from build123d import *

# Parameters (mm, degrees)
EXTRUDE_1_DEPTH     = 22.7
CUT_EXTRUDE_1_DEPTH = 1.2
SKETCH_3_R          = 1.25
SKETCH_3_W          = 8
SKETCH_3_H          = 6
CUT_EXTRUDE_2_DEPTH = 5
SKETCH_4_R          = 0.75
CUT_EXTRUDE_3_DEPTH = 5


with BuildPart() as part:
    # 草图1 → 凸台-拉伸1 (new body)
    with BuildSketch(Plane.XY):
        with BuildLine():
            Line((1.5, 0), (26.5, 0))
            ThreePointArc((26.5, 0), (27.560660172, 0.439339828), (28, 1.5))
            Line((28, 1.5), (28, 12.1))
            ThreePointArc((28, 12.1), (27.560660172, 13.160660172), (26.5, 13.6))
            Line((26.5, 13.6), (1.5, 13.6))
            ThreePointArc((1.5, 13.6), (0.439339828, 13.160660172), (0, 12.1))
            Line((0, 12.1), (0, 1.5))
            ThreePointArc((0, 1.5), (0.439339828, 0.439339828), (1.5, 0))
        make_face()
    extrude(amount=EXTRUDE_1_DEPTH)

    # 草图2 → 切除-拉伸1 (cut)
    with BuildSketch(Plane.XY.offset(22.7)):
        with BuildLine():
            ThreePointArc((0, 6.800000018), (1.991673894, 11.608326118), (6.8, 13.6))
            Line((6.8, 13.6), (1.5, 13.6))
            ThreePointArc((1.5, 13.6), (0.439339828, 13.160660172), (0, 12.1))
            Line((0, 12.1), (0, 6.800000018))
        make_face()
        with BuildLine():
            ThreePointArc((6.8, 0), (1.991673882, 1.991673894), (0, 6.800000018))
            Line((0, 6.800000018), (0, 1.5))
            ThreePointArc((0, 1.5), (0.439339828, 0.439339828), (1.5, 0))
            Line((1.5, 0), (6.8, 0))
        make_face()
        with BuildLine():
            Line((28, 1.5), (28, 6.8))
            ThreePointArc((28, 6.8), (26.008326112, 1.991673888), (21.2, 0))
            Line((21.2, 0), (26.5, 0))
            ThreePointArc((26.5, 0), (27.560660172, 0.439339828), (28, 1.5))
        make_face()
        with BuildLine():
            Line((26.5, 13.6), (21.2, 13.6))
            ThreePointArc((21.2, 13.6), (26.008326112, 11.608326112), (28, 6.8))
            Line((28, 6.8), (28, 12.1))
            ThreePointArc((28, 12.1), (27.560660172, 13.160660172), (26.5, 13.6))
        make_face()
    extrude(amount=-CUT_EXTRUDE_1_DEPTH, mode=Mode.SUBTRACT)

    # 草图3 → 切除-拉伸2 (cut)
    with BuildSketch(Plane(origin=(0, 0, 0), x_dir=(-1, 0, 0), z_dir=(0, 0, -1))):
        with Locations((-24.8, 6.8)):
            Circle(SKETCH_3_R)
        with Locations((-3.2, 6.8)):
            Circle(SKETCH_3_R)
        with Locations((-14, 6.8)):
            Rectangle(SKETCH_3_W, SKETCH_3_H)
    extrude(amount=-CUT_EXTRUDE_2_DEPTH, mode=Mode.SUBTRACT)

    # 草图4 → 切除-拉伸3 (cut)
    with BuildSketch(Plane.XZ):
        with Locations((24.8, 11.6)):
            Circle(SKETCH_4_R)
        with Locations((3.2, 11.6)):
            Circle(SKETCH_4_R)
    extrude(amount=-CUT_EXTRUDE_3_DEPTH, mode=Mode.SUBTRACT)


solid = part.part
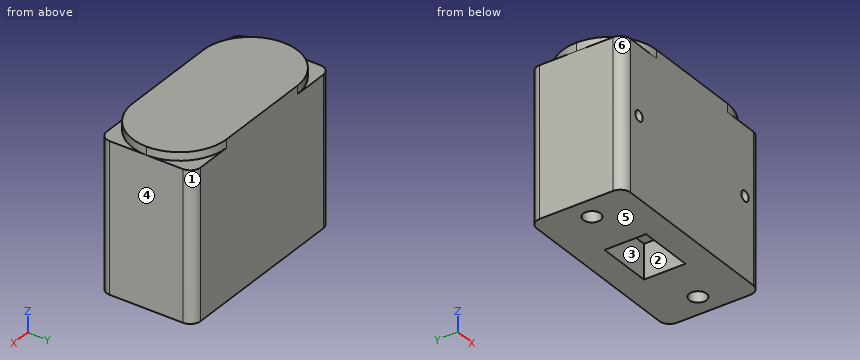
The listing builds one solid part. Answer for the finished solid, in the listing's coordinates (mm). Face numbers are marked on the shaded views. A direction names the side the tool comes from. Coordinates: 2 decimals unless noted, no trailing zeros. Write each loop counter-clockwise with the first axis right and the second up, starting at its lowest first coordinate (ties: lowest second). Pieces come first, ordered by that corner, then holes. Notation, with made-up numbers: (41, 36) - (76, 36) arc R23 cw to (76, 50) - close; hole circle Ø3 at (-6.5, 67.5). An arc over 180 degrees is marked (long way). Put each result on its own line as item: value.
1. The part is cut by section B-B on z = 11.6. Give the vertices of the cut face in (x, y).
Answer sheet:
outline: (0, 1.5) arc R1.5 ccw to (1.5, 0) - (2.45, 0) - (2.45, 5) - (3.95, 5) - (3.95, 0) - (24.05, 0) - (24.05, 5) - (25.55, 5) - (25.55, 0) - (26.5, 0) arc R1.5 ccw to (28, 1.5) - (28, 12.1) arc R1.5 ccw to (26.5, 13.6) - (1.5, 13.6) arc R1.5 ccw to (0, 12.1) - close
2. Determine the mould class of the marked faces 3, 4, 5 and 6 for opening direction X: pulls with the +X half, pulls with the -X half, needs draft (parallel to the pull), parting line crosses it, or undercut.
Answer sheet:
face 3: undercut
face 4: pulls with the +X half
face 5: needs draft
face 6: pulls with the -X half
3. The part is cut by section D-D on x = 3.2. Give the vertices of the cut face in (y, z), plus the area to 3 significant figures.
Answer sheet:
outline: (0, 0) - (5.55, 0) - (5.55, 5) - (8.05, 5) - (8.05, 0) - (13.6, 0) - (13.6, 21.5) - (12.57, 21.5) - (12.57, 22.7) - (1.03, 22.7) - (1.03, 21.5) - (0, 21.5) - (0, 12.35) - (5, 12.35) - (5, 10.85) - (0, 10.85) - close
area: 286 mm^2
4. Find the intervals of material crossed by line 1 along Z through (x, y) = (24.8, 2.25); line 2 along Y through (x, z) = (24.8, 2.45); line 3 along X through (y, z) = (12.25, 16.5), in increasing order. Write a range as from..to.
Answer sheet:
line 1: z = 0..10.85, 12.35..22.7
line 2: y = 0..5.55, 8.05..13.6
line 3: x = 0.01..27.99
5. A tool of negligible diameter and unlimited length cuts with its end or side. For the marked faces 1 and 2, from which of +Z, -Z, +X, -X, +Y, -Y can it reach the whole face along a straight path? Write none if from no direction.
Answer sheet:
face 1: +Z, -Z, +X, +Y
face 2: -Z
6. The part is cut by section A-A on x = 13.25. Give the vertices of the cut face in (y, z).
Answer sheet:
outline: (0, 0) - (3.8, 0) - (3.8, 5) - (9.8, 5) - (9.8, 0) - (13.6, 0) - (13.6, 22.7) - (0, 22.7) - close
7. A flat-ended cylindrical pin translates along its axis: pin 1 Ø2 at (x, y) = (24.8, 6.8) entering from -Z. Find the tip coordinate at first contact, or state that the pin passes through.
Answer sheet:
pin 1: stops at z = 5
